```python
from build123d import *

# Parameters (mm, degrees)
EXTRUDE_1_DEPTH = 3


with BuildPart() as part:
    # 草图1 → 凸台-拉伸1 (new body)
    with BuildSketch(Plane(origin=(0, 0, 0), x_dir=(1, 0, 0), z_dir=(0, 1, 0))):
        with BuildLine():
            Line((-35.122340396, 46.844577244), (40.579802215, 46.844577244))
            ThreePointArc((40.579802215, 46.844577244), (41.994015777, 46.258790806), (42.579802215, 44.844577244))
            Line((42.579802215, 44.844577244), (42.579802215, -28.502662655))
            ThreePointArc((42.579802215, -28.502662655), (41.994015777, -29.916876218), (40.579802215, -30.502662655))
            Line((40.579802215, -30.502662655), (-35.122340396, -30.502662655))
            ThreePointArc((-35.122340396, -30.502662655), (-36.536553959, -29.916876218), (-37.122340396, -28.502662655))
            Line((-37.122340396, -28.502662655), (-37.122340396, 44.844577244))
            ThreePointArc((-37.122340396, 44.844577244), (-36.536553959, 46.258790806), (-35.122340396, 46.844577244))
        make_face()
        Polygon((-28.122340396, 20.655786491), (-28.122340396, 38.844577244), (33.579802215, 38.844577244), (33.579802215, 20.655786491), (34.579802215, 20.655786491), (34.579802215, -22.502662655), (-29.122340396, -22.502662655), (-29.122340396, 20.655786491), align=None, mode=Mode.SUBTRACT)
    extrude(amount=EXTRUDE_1_DEPTH)


solid = part.part
```
Build history of the part. All positions in model axes, mm. A direction names the side the tool comes from. Round coordinates to 2 decimals unless told otherwise and drop trailing zeros. Write each loop counter-clockwise with the first axis right and the second up, starting at its lowest first coordinate (ties: lowest second). Pieces come first, ordered by that corner, then holes.
1) Band-saw the part on A-A, the plane z = -12. List the corners of the cut face in (x, y).
2) 3-axis set-ups, long thin cutter, end or side, ignore diameter. For faces 1 (the flat face through (42.58, 1, -9)), 2 (the flat face through (34.58, 1, 1)): which of +Z, -Z, +X, -X, +Y, -Y reach the whole face in a straight line?
3) Mould opens along Z. For faces 3 (the flat face through (-37.122, 1, -8)), 4 (the flat face through (3, 1, 22.503)), 5 (the cylindrical face through (-36.552, 1.479, -46.243)) say: +Z half, -Z half, draft (parallel to the pull), parting line (faces both ways), or undercut.
4) Band-saw the part on C-C, the plane y = 2.2. List the corners of the cut face in (x, z).
5) Band-saw the part on B-B, the plane x = -2. List the corners of the cut face in (y, z).
6) Drill centre lines: probe 1 along X at (y, z) = (1.6, -24); probe 2 along Z at (x, y) = (23, 1.85); probe 3 along X at (y, z) = (1.1, -19). Where is each one in solid material? Low to high.
Ans:
1. outline: (-37.12, 0) - (-29.12, 0) - (-29.12, 3) - (-37.12, 3) - close; (34.58, 0) - (42.58, 0) - (42.58, 3) - (34.58, 3) - close
2. face 1: +Z, -Z, +X, +Y, -Y
2. face 2: +Y, -Y
3. face 3: draft
3. face 4: undercut
3. face 5: -Z half
4. outline: (-37.12, -44.84) arc R2 ccw to (-35.12, -46.84) - (40.58, -46.84) arc R2 ccw to (42.58, -44.84) - (42.58, 28.5) arc R2 ccw to (40.58, 30.5) - (-35.12, 30.5) arc R2 ccw to (-37.12, 28.5) - close; hole (-29.12, -20.66) - (-28.12, -20.66) - (-28.12, -38.84) - (33.58, -38.84) - (33.58, -20.66) - (34.58, -20.66) - (34.58, 22.5) - (-29.12, 22.5) - close
5. outline: (0, -46.84) - (3, -46.84) - (3, -38.84) - (0, -38.84) - close; (0, 22.5) - (3, 22.5) - (3, 30.5) - (0, 30.5) - close
6. probe 1: x = -37.12 to -28.12, 33.58 to 42.58
6. probe 2: z = -46.84 to -38.84, 22.5 to 30.5
6. probe 3: x = -37.12 to -29.12, 34.58 to 42.58
